Part print with two shaded views. Sizes in mm from the minimum x, y, z corner. A direction names the side the tool comes from. Round coordinates to 2 decimals unless told otherwise and drop trailing zeros. Write each loop counter-clockwise with the first axis right and the second up, starting at its lowest first coordinate (ties: lowest second). Pieces come first, ordered by that corner, then holes. Notation, with made-up numbers: (27.25, 47.25) - (79.25, 47.25) arc R36 cw to (79.25, 85.25) - close; hole circle Ø8 at (83, 47.25). An arc over 180 degrees is marked (long way). Answer as a JSON object with one key per item and string values. Group by question number.
Item 1: Probe line 1 (X direction, y = 10.25, z = 4.5) (1 decimal); line 2 (X direction, y = 7.25, z = 10.25) (1 decimal); line 3 (Z direction, x = 5.5, y = 12.25). List the from-to ranges inside material, lowest first. Write a range as from..to.
Item 2: Flat gauge pins, fed straight in: pin 1 (4 mm diameter, centred on x = 13.5, z = 2, fed in from +Y); pin 2 (1 mm diameter, centred on x = 9.5, y = 4, fed in from -Z); pin 3 (5 mm diameter, centred on x = 3, z = 2.5, fed in from -Y) (1 decimal). Where does each tip first touch, or does it go through?
Item 3: Slice it at B-B, the plane z = 8.75. List the corners of the cut face in (x, y), then the cut area to 3 significant figures.
Item 4: Two-plate mould, pull along X, no slides. Class the marked faces 1, 2 and 3: +X half, -X half, draft (parallel to the pull), parting line (faces both ways), or undercut.
Item 5: Which spindle directions (+Z, -Z, +X, -X, +Y, -Y) get a long thin tool onto all of the face, cutting with end or side? Do the marked faces 4 and 5. Say none if no direction does.
Item 6: Slice it at A-A, the plane z = 1.75. List the corners of the cut face in (x, y).
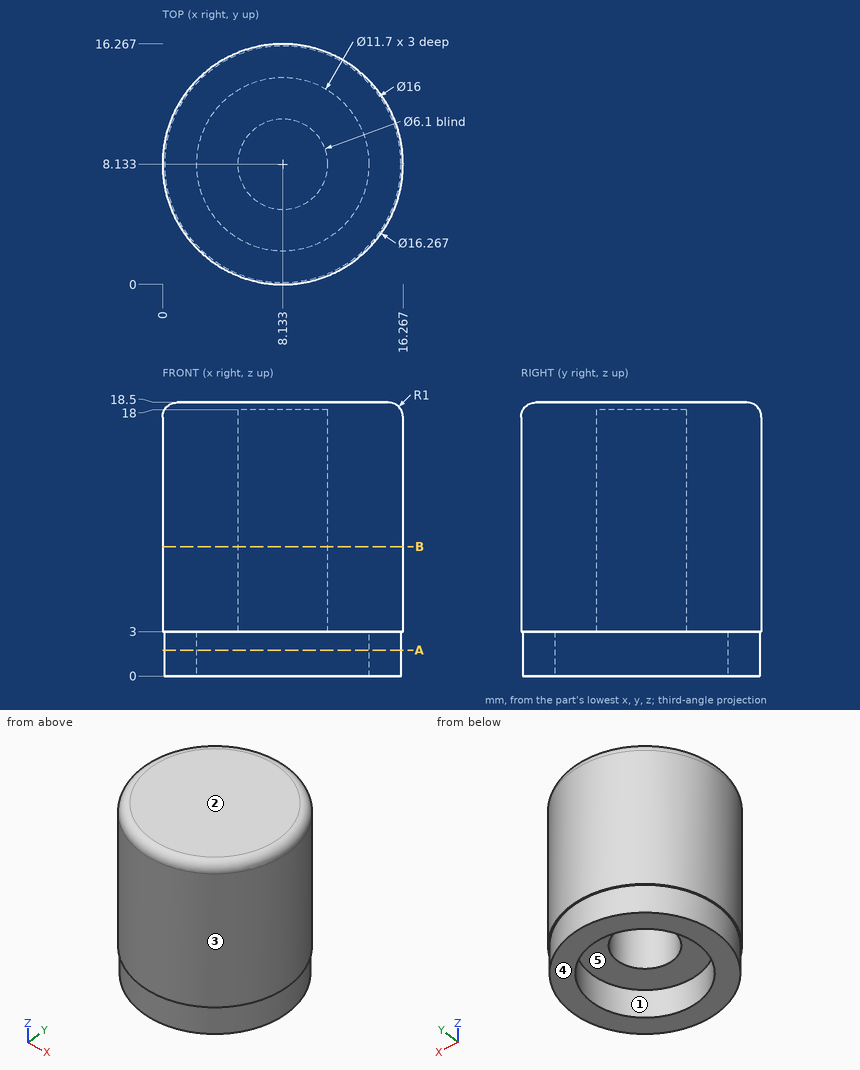
Geometry says:
{
 "1": {"line 1": "x = 0.3..5.9, 10.3..16", "line 2": "x = 0..5.2, 11.1..16.2", "line 3": "z = 3..18.5"},
 "2": {"pin 1": "stops at y = 15.41", "pin 2": "stops at z = 3", "pin 3": "stops at y = 0.5"},
 "3": {"outline": "circle Ø16.27 at (8.13, 8.13); hole circle Ø6.1 at (8.13, 8.13)", "area": "179 mm^2"},
 "4": {"face 1": "undercut", "face 2": "draft", "face 3": "parting line"},
 "5": {"face 4": "-Z, +X, -X, +Y, -Y", "face 5": "-Z"},
 "6": {"outline": "circle Ø16 at (8.13, 8.13); hole circle Ø11.7 at (8.13, 8.13)"}
}
